Can you work these out from the drawing? Everything is in mm from the part's minimum corner. A direction names the side the tool comes from. Round coordinates to 2 decimals unless told otherwise and drop trailing zeros. Loops run counter-clockwise (first coordinate to the right, second up) from the corner with the lowest first, then second, coordinate; pieces in that order, holes last. Notation, with made-up numbers: (-26.5, 3.5) -> (27.5, 3.5) arc R19 cw to (27.5, 20.5) -> close; hole circle Ø7 at (-2, -1). An arc over 180 degrees is marked (long way). One line per item, written item: value.
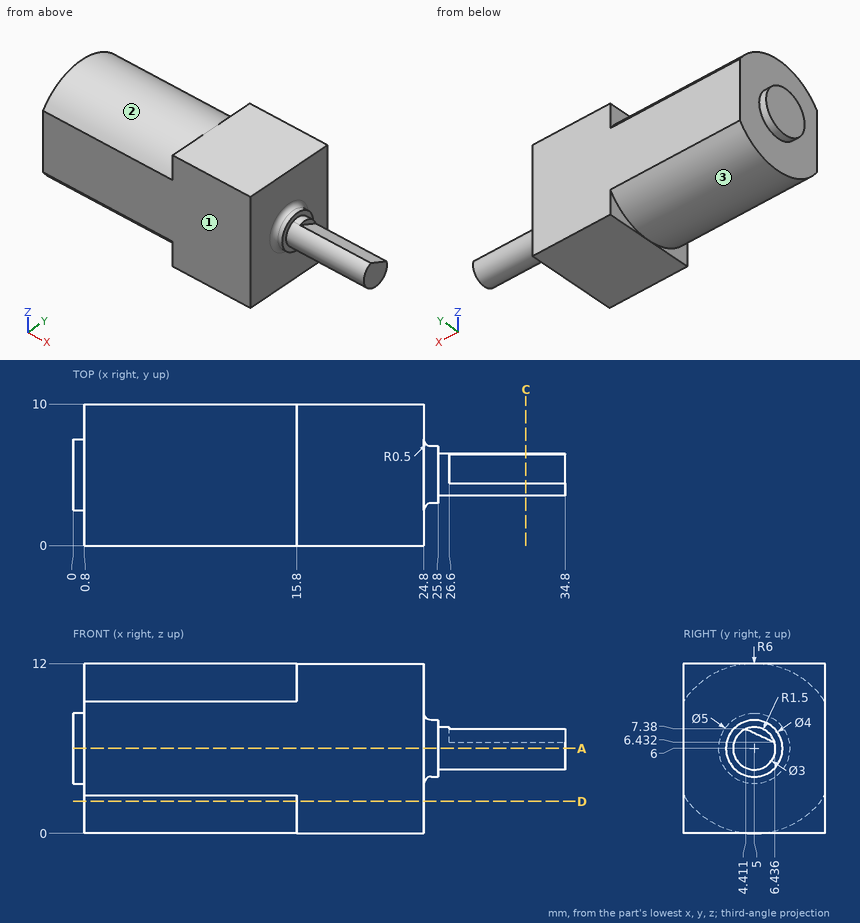
Item 1: For the marked faces 1, 2 and 3, which set-ups out of +Z, -Z, +X, -X, +Y, -Y let a thin tool reach every point of the face, with its end or its side?
Output:
face 1: +Z, -Z, +X, -X, -Y
face 2: +Z, -X
face 3: -Z, -X
Item 2: If we section it at D-D on z = 2.25: List the corners of the cut face in (x, y) for me.
Output:
outline: (0.8, 0.32) -> (15.8, 0.32) -> (15.8, 0) -> (24.8, 0) -> (24.8, 10) -> (15.8, 10) -> (15.8, 9.68) -> (0.8, 9.68) -> close
Item 3: Will these pins go through, and if not, where does the flat tip stop? pin 1 Ø3 at (y, z) = (5.5, 10.5) entering from -X; pin 2 Ø1 at (x, y) = (3.5, 2) entering from +Z (1 decimal); pin 3 Ø1.5 at (x, z) = (6, 10.5) entering from +Y (1 decimal).
Output:
pin 1: stops at x = 0.8
pin 2: stops at z = 11.5
pin 3: stops at y = 9.7
Item 4: I need wall thicknesses on line 1 (X direction, y = 3.25, z = 8.5); line 2 (Z direction, x = 9.5, y = 3.5); line 3 (Y direction, x = 27.5, z = 5.75). Which ranges of each line are inside material? Lowest first, please. Write a range as from..to.
Output:
line 1: x = 0.8..24.8
line 2: z = 0.19..11.81
line 3: y = 3.52..6.48
Item 5: If we section it at C-C on x = 32: List the corners of the cut face in (y, z) for me.
Output:
outline: (4.41, 7.38) arc R1.5 ccw (long way) to (6.44, 6.43) -> close
Item 6: If we section it at A-A on z = 6: List the corners of the cut face in (x, y) for me.
Output:
outline: (0, 2.5) -> (0.8, 2.5) -> (0.8, 0) -> (24.8, 0) -> (24.8, 2.5) arc R0.5 cw to (25.3, 3) -> (25.8, 3) -> (25.8, 3.5) -> (34.8, 3.5) -> (34.8, 6.5) -> (25.8, 6.5) -> (25.8, 7) -> (25.3, 7) arc R0.5 cw to (24.8, 7.5) -> (24.8, 10) -> (0.8, 10) -> (0.8, 7.5) -> (0, 7.5) -> close
